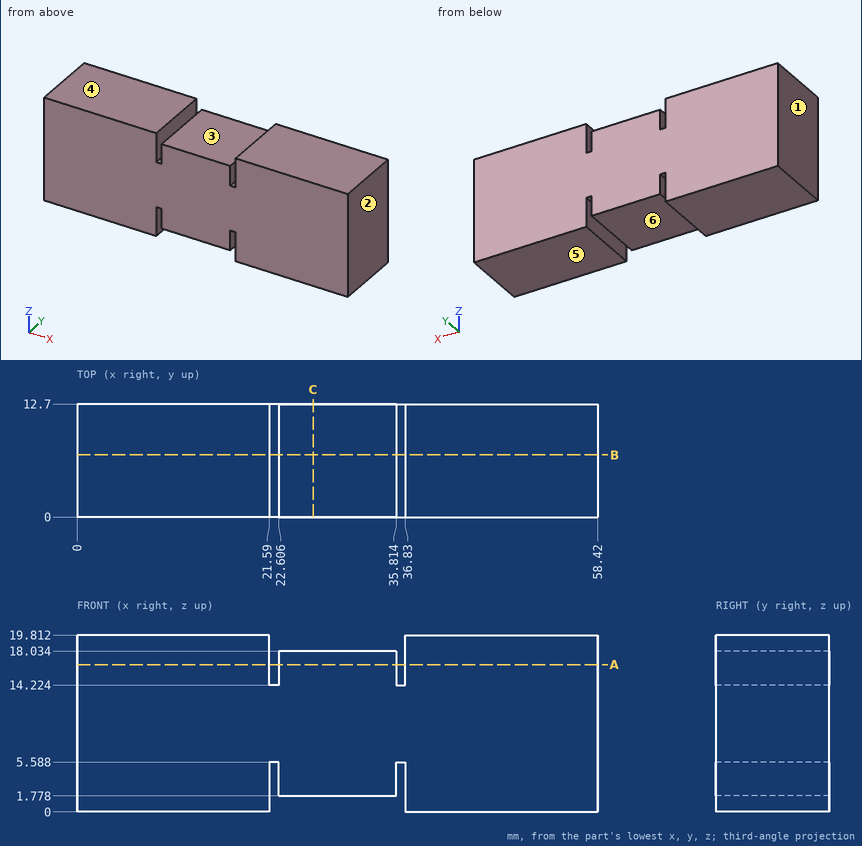
Job drawing, mm, ordinate dimensions from the low corner. One solid piece. A direction names the side the tool comes from. Coordinates: 2 decimals unless noted, no trailing zeros. Order: outer loops, then holes, each group sorted by start corner. A loop starts at its lowest first (then second) coordinate and runs counter-clockwise, first axis right, second up. Notation, with made-up numbers: M 79,-39 L 124,-39 A33 ccw 124,-7 Z; hole C -15.75,-7 d10. An arc over 180 degrees is marked long. Return JSON: item names as keys, results as strings.
1. Saw through at B-B (y = 7). Give the cut face in (x, z).
Ans:
{"outline": "M 0,0 L 21.59,0 L 21.59,5.59 L 22.61,5.59 L 22.61,1.78 L 35.81,1.78 L 35.81,5.59 L 36.83,5.59 L 36.83,0 L 58.42,0 L 58.42,19.81 L 36.83,19.81 L 36.83,14.22 L 35.81,14.22 L 35.81,18.03 L 22.61,18.03 L 22.61,14.22 L 21.59,14.22 L 21.59,19.81 L 0,19.81 Z"}
2. Saw through at A-A (z = 16.5). Give the cut face in (x, y).
Ans:
{"outline": "M 0,0 L 21.59,0 L 21.59,12.7 L 0,12.7 Z; M 22.61,0 L 35.81,0 L 35.81,12.7 L 22.61,12.7 Z; M 36.83,0 L 58.42,0 L 58.42,12.7 L 36.83,12.7 Z"}
3. Drill centre lines: probe 1 along X at (y, z) = (2.5, 17.25); probe 2 along X at (y, z) = (6, 1.5); probe 3 along Z at (x, y) = (28.5, 5.5). Where is each one in solid material? Low to high.
Ans:
{"probe 1": "0 to 21.59, 22.61 to 35.81, 36.83 to 58.42", "probe 2": "0 to 21.59, 36.83 to 58.42", "probe 3": "1.78 to 18.03"}
4. Flat gauge pins, fed straight in: pin 1 (6.5 mm diameter, centred on x = 29.5, y = 7.5, fed in from +Z); pin 2 (1.5 mm diameter, centred on x = 31, y = 10, fed in from -Z). Where does each tip first touch, or does it go through?
Ans:
{"pin 1": "z = 18.03", "pin 2": "z = 1.78"}
5. Saw through at C-C (x = 26.5). Give the cut face in (y, z), and give its area (3 significant figures).
Ans:
{"outline": "M 0,1.78 L 12.7,1.78 L 12.7,18.03 L 0,18.03 Z", "area": "206 mm^2"}
6. Tool access for the marked faces 5 and 6: list every direction of +Z, -Z, +X, -X, +Y, -Y with a clear straight run to the whole face (end or side of a thin tool).
Ans:
{"face 5": "-Z, +X, -X, +Y, -Y", "face 6": "-Z, +Y, -Y"}
7. Pull direction X, two halves, no side cores. Call the marked faces 1, 2, 3 and 4: +X half, -X half, draft (parallel to the pull), parting line (faces both ways), or undercut.
Ans:
{"face 1": "-X half", "face 2": "+X half", "face 3": "undercut", "face 4": "draft"}
